Check sheet for the modelled part. Datum: model origin and axes. Units: mm. A direction names the side the tool comes from. Give positions to 0.01 mm unless a question says otherwise; leave off trailing zeros. Write each loop counter-clockwise with the first axis right and the second up, starting at its lowest first coordinate (ties: lowest second). Pieces come first, ordered by that corner, then holes. Notation, with made-up numbers: M -34,38.5 L 2,38.5 A25 ccw 2,57.5 Z; hole C -30.5,-15 d2. An arc over 180 degrees is marked long. Write item = value, one per line. Start each with the question number.
1) Access from +Z, -Z, +X, -X, +Y, -Y to the whole of each face (thin tool, end or side, straight path). Record for faces 4 (the flat face through (3, 3.175, -3)), 5 (the flat face through (-5, 1.588, 1)).
2) Mould release check, pull along Z, two halves, no side actions. Record for faces 1 (the flat face through (3, -3.175, 2)), 2 (the cylindrical face through (2.9, -0.83, -3.78)), 3 (the cylindrical face through (1.93, 0.04, -2.52)): released by +Z, released by -Z, zero draft, split by the parting line, or undercut.
3) Go/stop test with flat-tipped pins: pin 1 (3 mm diameter, centred on x = -3.5, y = -2, fed in from +Z); pin 2 (4 mm diameter, centred on x = 5, z = 4.5, fed in from -Y) (3 decimals). Record where each tip stops, or that it passes through.
4) Cross-section at D-D, the plane z = 3.75. Record the cut outline in (x, y) (1 decimal).
5) Cross-section at C-C, the plane y = 2.75. Record the cut outline in (x, z) (3 decimals), plus the area to 3 significant figures.
6) Scan lines: line 1 along X through (y, z) = (1.4, 0) (1 decimal); line 2 along Y through (x, z) = (-3.5, 5) (1 decimal); line 3 along Z through (x, y) = (-0.5, -0.25). Record each from-to range of solid material in increasing order. Write a range as [from, to].
```python
from build123d import *

# Parameters (mm, degrees)
CHAMFER1_SIZE = 0.254


with BuildPart() as part:
    # Sketch1 → Revolve1 (revolve)
    with BuildSketch(Plane.XY, mode=Mode.PRIVATE) as revolve1_sk:
        Polygon((-3.175, 3.175), (-6.35, 3.175), (-6.35, 1.5875), (-4.7625, 1.5875), (-4.7625, -3.175), (-3.175, -3.175), align=None)
    revolve(revolve1_sk.sketch.rotate(Axis((0, 6.35, 0), (0, -1, 0)), 270), axis=Axis((0, 6.35, 0), (0, -1, 0)))

    # Chamfer1
    chamfer1_edges = [part.edges().sort_by_distance(p)[0] for p in [
        (0, -3.175, -3.175),
        (0, 3.175, -3.175),
    ]]
    chamfer(chamfer1_edges, length=CHAMFER1_SIZE)


solid = part.part
```
Reply:
q1.face_4 = +Z, -Z, +X, -X, +Y
q1.face_5 = -Y
q2.face_1 = zero draft
q2.face_2 = split by the parting line
q2.face_3 = undercut
q3.pin_1 = 4.32
q3.pin_2 = -3.175
q4.outline = M -5.1,1.6 L -2.9,1.6 L -2.9,-3.2 L 2.9,-3.2 L 2.9,1.6 L 5.1,1.6 L 5.1,3.2 L -5.1,3.2 Z
q5.outline = C 0,0 d12.7; hole C 0,0 d6.35
q5.area = 95.0 mm2
q6.line_1 = [-4.8, -3.2], [3.2, 4.8]
q6.line_2 = [1.6, 3.2]
q6.line_3 = [-4.74, -3.14], [3.14, 4.74]
